```python
from build123d import *

# Parameters (mm, degrees)
F0_W     = 1866
F0_H     = 885
F1_DEPTH = 25
F0_H_2   = 30
F0_W_2   = 360
F0_H_3   = 380
F2_DEPTH = 20
F3_DEPTH = 15
F4_DEPTH = 30


with BuildPart() as f1:
    # F0 (on Top) → F1 (new body)
    with BuildSketch(Plane.XY):
        with Locations((933, 442.5)):
            Rectangle(F0_W, F0_H)
        Polygon((573, 50), (213, 50), (213, 430), (213, 810), (573, 810), (573, 430), (933, 430), (1293, 430), (1293, 810), (1653, 810), (1653, 430), (1653, 50), (1293, 50), (933, 50), align=None, mode=Mode.SUBTRACT)
    extrude(amount=F1_DEPTH)

    # F0 (on Top) → F2 (join)
    with BuildSketch(Plane.XY):
        with Locations((933, 900)):
            Rectangle(F0_W, F0_H_2)
        with Locations((393, 620)):
            Rectangle(F0_W_2, F0_H_3)
        with Locations((753, 240)):
            Rectangle(F0_W_2, F0_H_3)
        with Locations((1473, 620)):
            Rectangle(F0_W_2, F0_H_3)
    extrude(amount=F2_DEPTH)

    # F0 (on Top) → F3 (join)
    with BuildSketch(Plane.XY):
        with Locations((1473, 240)):
            Rectangle(F0_W_2, F0_H_3)
        with Locations((393, 240)):
            Rectangle(F0_W_2, F0_H_3)
    extrude(amount=F3_DEPTH)

    # F0 (on Top) → F4 (join)
    with BuildSketch(Plane.XY):
        with Locations((1113, 240)):
            Rectangle(F0_W_2, F0_H_3)
    extrude(amount=F4_DEPTH)


solid = f1.part
```
For this review, take the finished solid that the model builds, in its own axes (mm). A direction names the side the tool comes from. Give positions to 0.01 mm unless a question says otherwise; leave off trailing zeros. Write each loop counter-clockwise with the first axis right and the second up, starting at its lowest first coordinate (ties: lowest second). Pieces come first, ordered by that corner, then holes. Notation, with made-up numbers: M -37.75,6 L 7.25,6 A13 ccw 7.25,22 Z; hole C 13.5,55.25 d4. An arc over 180 degrees is marked long. One line per item, written item: value.
1) Take a section at B-B, the plane x = 727. Write out the cut boundary in (y, z), then the cut area to 3 significant figures.
Results are:
outline: M 0,0 L 915,0 L 915,20 L 885,20 L 885,25 L 430,25 L 430,20 L 50,20 L 50,25 L 0,25 Z
area: 20,800 mm²
2) Take a section at A-A, the plane y = 124. Write out the cut boundary in (x, z).
Results are:
outline: M 0,0 L 1866,0 L 1866,25 L 1653,25 L 1653,15 L 1293,15 L 1293,30 L 933,30 L 933,20 L 573,20 L 573,15 L 213,15 L 213,25 L 0,25 Z
3) Take a section at D-D, the plane y = 596.5. Write out the cut boundary in (x, z), then the cut area to 4 significant figures.
Results are:
outline: M 0,0 L 1866,0 L 1866,25 L 1653,25 L 1653,20 L 1293,20 L 1293,25 L 573,25 L 573,20 L 213,20 L 213,25 L 0,25 Z
area: 43,050 mm²
4) For faces 3 (the flat face through (750, 243, 20)), 4 (the flat face through (920, 464, 0)), list the 3-axis set-ups (+Z, -Z, +X, -X, +Y, -Y) from which the entire face can be reached by the end or side of a thin tool; tool diameter is ignored.
Results are:
face 3: +Z
face 4: -Z, +X, -X, +Y, -Y
5) For P1, Ø4, axis at x = 407.5, y = 775.5, coming from the +Z side; P2, Ø5.5, axis at y = 617.5, z = 22.5, coming from the -X side; P3, Ø5.5, axis at x = 1189, z = 28.5, coming from the +Y side; P4, Ø10, axis at x = 1230.5, y = 436, coming from the +Z side, all flat-tipped, find the tip position at first contact; note any pin that passes through.
Results are:
P1: stops at z = 20
P2: stops at x = 0
P3: stops at y = 430
P4: stops at z = 25
6) The part is to be moulded in two halves that separate along X. For faces 1 (the flat face through (920, 547, 25)), 2 (the flat face through (1470, 243, 15)), say which applies: +X half, -X half, draft (parallel to the pull), parting line (faces both ways), or undercut.
Results are:
face 1: draft
face 2: undercut
7) For line 1 (X direction, y = 159.5, z = 24.5); line 2 (X direction, y = 255, z = 18); line 3 (Y direction, x = 1335, z = 15.5), list the stretches that pass through material, from the lowest coordinate up. Write a range as from..to.
Results are:
line 1: x = 0..213, 933..1293, 1653..1866
line 2: x = 0..213, 573..1293, 1653..1866
line 3: y = 0..50, 430..915
8) Take a section at C-C, the plane x = 1220.5. Write out the cut boundary in (y, z).
Results are:
outline: M 0,0 L 915,0 L 915,20 L 885,20 L 885,25 L 430,25 L 430,30 L 50,30 L 50,25 L 0,25 Z
